Here's how the part is built. I have some questions about the finished solid (model axes, mm). Face numbers are marked on the shaded views. A direction names the side the tool comes from. Round coordinates to 2 decimals unless told otherwise and drop trailing zeros. Order: outer loops, then holes, each group sorted by start corner. A loop starts at its lowest first (then second) coordinate and runs counter-clockwise, first axis right, second up. Notation, with made-up numbers: (-3, 17) -> (35, 17) arc R14 cw to (35, 27) -> close; hole circle Ø10 at (49.5, 89.25). An arc over 180 degrees is marked (long way). Use a Markdown table: item, result. Add a question column.
(1) I want a section at C-C, the plane x = 5.3. Give the number of separate pieces and of enclosed holes in the cut face, then the cut area to 3 significant figures.
(2) I want a section at A-A, the plane z = 0. Please give me the cut outline in (x, y).
(3) Thinking about a two-plate mould opening in Y: for the marked faces 1, 2 and 3, which applies, pulls with the +Y half, pulls with the -Y half, needs draft (parallel to the pull), parting line crosses it, or undercut?
(4) I want a section at D-D, the plane y = 6.5. Please give me the cut outline in (x, z).
(5) If I drill on probe 1 along Y at (x, z) = (2.65, 0); probe 2 along Z at (x, y) = (5.2, -11); probe 3 along Z at (x, y) = (0.4, 13.5), over which ranges is the centre line in solid material (lowest first)?
(6) I'm going to push flat-ended pins straight in: P1, Ø1.5, axis at x = 1, y = -4.5, coming from the -Z side; P2, Ø1, axis at x = 2, y = -10.5, coming from the +Z side; P3, Ø1, axis at x = 3, y = 11, coming from the +Z side. Where does each tip first touch, or does it pass through?
(7) On a 3-axis mill with a long thin cutter (end or side, diameter ignored), from which of +Z, -Z, +X, -X, +Y, -Y can I reach the whole of each face in a straight line? I mean the marked faces 4, 5 and 6. Say none if no direction works.
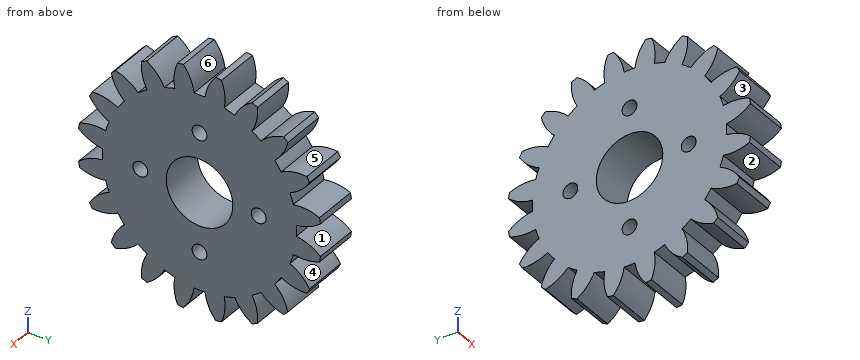
from build123d import *

# Parameters (mm, degrees)
BASPROSKE_W             = 6
BASPROSKE_H             = 16.5
TOOTHCUT_DEPTH          = 25.093567606
TEETHCUTS_COUNT         = 20
TEETHCUTS_ANGLE         = 342
BORSKE_R                = 4.5
BORE_DEPTH              = 50.0000508
ESQUISSE2_R             = 1
ENL_V_MAT_EXTRU_1_DEPTH = 6


with BuildPart() as part:
    # BasProSke → Base-Revolve (revolve)
    with BuildSketch(Plane(origin=(0, 0, 0), x_dir=(1, 0, 0), z_dir=(0, 1, 0)), mode=Mode.PRIVATE) as base_revolve_sk:
        with Locations((3, 8.25)):
            Rectangle(BASPROSKE_W, BASPROSKE_H)
    revolve(base_revolve_sk.sketch.rotate(Axis((-10, 0, 0), (1, 0, 0)), 180), axis=Axis((-10, 0, 0), (1, 0, 0)))

    # TooCutSke → ToothCut (cut, through all)
    with BuildSketch(Plane(origin=(0, 0, 0), x_dir=(0, 0, -1), z_dir=(1, 0, 0))):
        with BuildLine():
            ThreePointArc((0.74381438, 13.102904875), (0, 13.124), (-0.74381438, 13.102904875))
            ThreePointArc((-0.74381438, 13.102904875), (-1.226473103, 14.852072512), (-2.209965745, 16.376962373))
            ThreePointArc((-2.209965745, 16.376962373), (0, 16.5254), (2.209965745, 16.376962373))
            ThreePointArc((2.209965745, 16.376962373), (1.226473103, 14.852072512), (0.74381438, 13.102904875))
        make_face()
    toothcut = extrude(amount=TOOTHCUT_DEPTH, mode=Mode.SUBTRACT)

    # TeethCuts: ToothCut ×20 about axis
    teethcuts_axis = Axis((-10, 0, 0), (1, 0, 0))
    for i in range(1, TEETHCUTS_COUNT):
        add(toothcut.rotate(teethcuts_axis, i * TEETHCUTS_ANGLE / (TEETHCUTS_COUNT - 1)), mode=Mode.SUBTRACT)

    # BorSke → Bore (cut, symmetric)
    with BuildSketch(Plane(origin=(0, 0, 0), x_dir=(0, 0, -1), z_dir=(1, 0, 0))):
        with Locations(Location((0, 0, 0), (0, 0, 180))):
            Circle(BORSKE_R)
    extrude(amount=BORE_DEPTH, both=True, mode=Mode.SUBTRACT)

    # Esquisse2 → Enlèv. mat.-Extru.1 (cut)
    with BuildSketch(Plane(origin=(6, 0, 0), x_dir=(0, 0, -1), z_dir=(1, 0, 0))):
        with Locations((0, 8)):
            Circle(ESQUISSE2_R)
        with Locations((8, 0)):
            Circle(ESQUISSE2_R)
        with Locations((0, -8)):
            Circle(ESQUISSE2_R)
        with Locations((-8, 0)):
            Circle(ESQUISSE2_R)
    extrude(amount=-ENL_V_MAT_EXTRU_1_DEPTH, mode=Mode.SUBTRACT)


solid = part.part
Taken from the geometry:
| question | item | result |
|---|---|---|
| 1 | separate pieces | 1 |
| 1 | enclosed holes | 5 |
| 1 | area | 606 mm2 |
| 2 | outline | (0, -13.12) -> (6, -13.12) -> (6, -9) -> (0, -9) -> close; (0, -7) -> (6, -7) -> (6, -4.5) -> (0, -4.5) -> close; (0, 4.5) -> (6, 4.5) -> (6, 7) -> (0, 7) -> close; (0, 9) -> (6, 9) -> (6, 13.12) -> (0, 13.12) -> close |
| 3 | face 1 | pulls with the +Y half |
| 3 | face 2 | undercut |
| 3 | face 3 | pulls with the -Y half |
| 4 | outline | (0, -14.44) -> (6, -14.44) -> (6, 14.44) -> (0, 14.44) -> close |
| 5 | probe 1 | y = -13.12 to -9, -7 to -4.5, 4.5 to 7, 9 to 13.12 |
| 5 | probe 2 | z = -11.84 to -9.26, -7.16 to 7.16, 9.26 to 11.84 |
| 5 | probe 3 | z = -7.85 to -5.55, -3.45 to -0.8, 0.8 to 3.45, 5.55 to 7.85 |
| 6 | P1 | stops at z = -13.1 |
| 6 | P2 | stops at z = 11.84 |
| 6 | P3 | stops at z = 11.94 |
| 7 | face 4 | +X, -X, +Y |
| 7 | face 5 | +X, -X |
| 7 | face 6 | +Z, +X, -X |
